from build123d import *

# Parameters (mm, degrees)
ESBO_O1_W                = 103
ESBO_O1_H                = 15
RESSALTO_EXTRUS_O1_DEPTH = 2
ESBO_O2_W                = 2
ESBO_O2_H                = 15
RESSALTO_EXTRUS_O2_DEPTH = 42
ESBO_O4_R                = 1.55
CORTE_EXTRUS_O1_DEPTH    = 2
FILETE1_R                = 1


with BuildPart() as part:
    # Esboço1 → Ressalto-extrusão1 (new body)
    with BuildSketch(Plane(origin=(0, 0, 0), x_dir=(1, 0, 0), z_dir=(0, 1, 0))):
        Rectangle(ESBO_O1_W, ESBO_O1_H)
    extrude(amount=-RESSALTO_EXTRUS_O1_DEPTH)

    # Esboço2 → Ressalto-extrusão2 (add)
    with BuildSketch(Plane(origin=(0, 0, 0), x_dir=(1, 0, 0), z_dir=(0, 1, 0))):
        with Locations((-50.5, 0)):
            Rectangle(ESBO_O2_W, ESBO_O2_H)
        with Locations((50.5, 0)):
            Rectangle(ESBO_O2_W, ESBO_O2_H)
    extrude(amount=RESSALTO_EXTRUS_O2_DEPTH)

    # Esboço4 → Corte-extrusão1 (cut)
    with BuildSketch(Plane(origin=(0, 0, 0), x_dir=(1, 0, 0), z_dir=(0, 1, 0))):
        with Locations(Location((24.75, 0, 0), (0, 0, 270))):
            Circle(ESBO_O4_R)
        with Locations(Location((-24.75, 0, 0), (0, 0, 90))):
            Circle(ESBO_O4_R)
    extrude(amount=-CORTE_EXTRUS_O1_DEPTH, mode=Mode.SUBTRACT)

    # Filete1
    filete1_edges = [part.edges().sort_by_distance(p)[0] for p in [
        (51.5, 20, 7.5),
        (-51.5, 20, 7.5),
    ]]
    fillet(filete1_edges, radius=FILETE1_R)


solid = part.part
CAD build for the part. Positions are in the model's coordinates, mm. A direction names the side the tool comes from. Give positions to 0.01 mm unless a question says otherwise; leave off trailing zeros. Loops run counter-clockwise (first coordinate to the right, second up) from the corner with the lowest first, then second, coordinate; pieces in that order, holes last. Notation, with made-up numbers: M 70,-25 L 119,-25 A29 ccw 119,0 Z; hole C 73,4 d2. An arc over 180 degrees is marked long. Answer in a Markdown table with one row per item. Add a question column.
Item 1: Probe probe 1 along X at (y, z) = (-0.9, 0); probe 2 along Z at (x, y) = (-24.75, -1); probe 3 along X at (y, z) = (10, -3.5). List the from-to ranges inside material, lowest first.
Item 2: Band-saw the part on C-C on y = 15. Give the cut face in (x, z), then the cut area to 3 significant figures.
Item 3: Band-saw the part on D-D on x = 20. Give the cut face in (y, z).
Item 4: Band-saw the part on A-A on z = 0. Give the cut face in (x, y).
Item 5: Drop flat-ended pins along their axis: P1, Ø6, axis at x = -8, z = -1, coming from the +Y side; P2, Ø3, axis at x = -24.75, z = 0, coming from the +Y side. Give the stop position or say it passes through.
Item 6: Band-saw the part on B-B on x = -24.75. Give the cut face in (y, z).
Item 7: Mould opens along X. For faces 3 (the face through (-51.5, 20, 0)), 4 (the face through (-1, -2, 0)), 5 (the face through (-26.287, -0.986, 0.202)) say: +X half, -X half, draft (parallel to the pull), parting line (faces both ways), or undercut.
Item 8: Tool access for faces 1 (the face through (-1, 0, 0)), 2 (the face through (-23, -1, -7.5)): list every direction of +Z, -Z, +X, -X, +Y, -Y with a clear straight run to the whole face (end or side of a thin tool).
Reply:
| question | item | result |
|---|---|---|
| 1 | probe 1 | x = -51.5 to -26.3, -23.2 to 23.2, 26.3 to 51.5 |
| 1 | probe 2 | z = -7.5 to -1.55, 1.55 to 7.5 |
| 1 | probe 3 | x = -51.5 to -49.5, 49.5 to 51.5 |
| 2 | outline | M -51.5,-7.5 L -49.5,-7.5 L -49.5,7.5 L -50.5,7.5 A1 ccw -51.5,6.5 Z; M 49.5,-7.5 L 51.5,-7.5 L 51.5,6.5 A1 ccw 50.5,7.5 L 49.5,7.5 Z |
| 2 | area | 59.6 mm^2 |
| 3 | outline | M -2,-7.5 L 0,-7.5 L 0,7.5 L -2,7.5 Z |
| 4 | outline | M -51.5,-2 L -26.3,-2 L -26.3,0 L -49.5,0 L -49.5,42 L -51.5,42 Z; M -23.2,-2 L 23.2,-2 L 23.2,0 L -23.2,0 Z; M 26.3,-2 L 51.5,-2 L 51.5,42 L 49.5,42 L 49.5,0 L 26.3,0 Z |
| 5 | P1 | stops at y = 0 |
| 5 | P2 | passes through |
| 6 | outline | M -2,-7.5 L 0,-7.5 L 0,-1.55 L -2,-1.55 Z; M -2,1.55 L 0,1.55 L 0,7.5 L -2,7.5 Z |
| 7 | face 3 | -X half |
| 7 | face 4 | draft |
| 7 | face 5 | undercut |
| 8 | face 1 | +Z, -Z, +Y |
| 8 | face 2 | -Z, +X, -X, +Y, -Y |
